CAD build for the part. Positions are in the model's coordinates, mm. A direction names the side the tool comes from. Give positions to 0.01 mm unless a question says otherwise; leave off trailing zeros. Write each loop counter-clockwise with the first axis right and the second up, starting at its lowest first coordinate (ties: lowest second). Pieces come first, ordered by that corner, then holes. Notation, with made-up numbers: (69.5, -9.75) -> (123.5, -9.75) arc R25 ccw to (123.5, 7.25) -> close; hole circle Ø8 at (82.25, 24.5). An arc over 180 degrees is marked (long way). Answer as a JSON object with one key per item and string values.
```python
from build123d import *

# Parameters (mm, degrees)
F0_R           = 9.525
F1_DEPTH       = 31.5468
F3_D           = 9.8044
F3_CBORE_D     = 11.9126
F3_CBORE_DEPTH = 29.0068
F4_R           = 6.9215
F5_DEPTH       = 6.6294
F6_SIZE2       = 1.5875
F6_SIZE        = 1.5875


with BuildPart() as f1:
    # F0 (on Front) → F1 (new body)
    with BuildSketch(Plane.XZ):
        Circle(F0_R)
    extrude(amount=F1_DEPTH)

    # F3 (through all)
    with Locations(Plane.XZ.offset(31.5468)):
        with Locations((0, 0)):
            CounterBoreHole(F3_D / 2, F3_CBORE_D / 2, F3_CBORE_DEPTH)

    # F4 (on face) → F5 (cut)
    with BuildSketch(Plane.XZ.offset(31.5468)):
        Circle(F4_R)
    extrude(amount=-F5_DEPTH, mode=Mode.SUBTRACT)

    # F6
    f6_edges = [f1.edges().sort_by_distance(p)[0] for p in [
        (-9.525, -31.5468, 0),
        (-9.525, 0, 0),
    ]]
    chamfer(f6_edges, length=F6_SIZE, length2=F6_SIZE2)


solid = f1.part
```
1) Slice it at B-B (x = 0). List the corners of the cut face in (y, z) (1 decimal), then the cut area to 3 significant figures.
Model answer:
{"outline": "(-31.5, -7.9) -> (-30, -9.5) -> (-1.6, -9.5) -> (0, -7.9) -> (0, -4.9) -> (-2.5, -4.9) -> (-2.5, -6) -> (-24.9, -6) -> (-24.9, -6.9) -> (-31.5, -6.9) -> close; (-31.5, 6.9) -> (-24.9, 6.9) -> (-24.9, 6) -> (-2.5, 6) -> (-2.5, 4.9) -> (0, 4.9) -> (0, 7.9) -> (-1.6, 9.5) -> (-30, 9.5) -> (-31.5, 7.9) -> close", "area": "213 mm2"}
2) 3-axis set-ups, long thin cutter, end or side, ignore diameter. For faces 1 (the cylindrical face through (3.721, -28.279, 5.836)), 2 (the flat face through (-2, -31.547, 7)): which of +Z, -Z, +X, -X, +Y, -Y reach the whole face in a straight line?
Model answer:
{"face 1": "-Y", "face 2": "+Z, -Z, +X, -X, -Y"}
3) Slice it at C-C (y = -18.5). List the corners of the cut face in (x, z) (3 decimals).
Model answer:
{"outline": "circle Ø19.05 at (0, 0); hole circle Ø11.913 at (0, 0)"}
4) Mould opens along X. For faces 3 (the cylindrical face through (-7.559, -15.575, -5.796)), 4 (the flat face through (-0.1, 0, -5.2)), 5 (the flat face through (2, -24.917, 6)) say: released by +X, released by -X, zero draft, split by the parting line, or undercut.
Model answer:
{"face 3": "split by the parting line", "face 4": "zero draft", "face 5": "undercut"}
5) Slice it at A-A (z = 0). List the corners of the cut face in (x, y) (1 decimal).
Model answer:
{"outline": "(-9.5, -30) -> (-7.9, -31.5) -> (-6.9, -31.5) -> (-6.9, -24.9) -> (-6, -24.9) -> (-6, -2.5) -> (-4.9, -2.5) -> (-4.9, 0) -> (-7.9, 0) -> (-9.5, -1.6) -> close; (4.9, -2.5) -> (6, -2.5) -> (6, -24.9) -> (6.9, -24.9) -> (6.9, -31.5) -> (7.9, -31.5) -> (9.5, -30) -> (9.5, -1.6) -> (7.9, 0) -> (4.9, 0) -> close"}
6) Wall check: probe 1 along Z at (x, y) = (0, -17.25) (3 decimals); probe 2 along Z at (x, y) = (0, -1.8) (3 decimals); probe 3 along Y at (x, z) = (-1.25, -6). Give the ranges that are in metal, low to high.
Model answer:
{"probe 1": "z = -9.525 to -5.956, 5.956 to 9.525", "probe 2": "z = -9.525 to -4.902, 4.902 to 9.525", "probe 3": "y = -24.92 to 0"}
7) Pin check, flat tips, straight feed: pin 1 (1 mm diameter, centred on x = -2, y = -5, fed in from -Z); pin 2 (10 mm diameter, centred on x = 7, y = -3.5, fed in from +Z); pin 3 (4 mm diameter, centred on y = -24.5, z = -6, fed in from -X); pin 4 (3.5 mm diameter, centred on x = -1.5, z = -1.5, fed in from -Y). Stop position of each tip, or through.
Model answer:
{"pin 1": "stops at z = -9.41", "pin 2": "stops at z = 9.31", "pin 3": "stops at x = -8.64", "pin 4": "passes through"}
